```python
from build123d import *

# Parameters (mm, degrees)
RESSALTO_EXTRUS_O1_DEPTH = 6


with BuildPart() as part:
    # Model → Ressalto-extrusão1 (new body)
    with BuildSketch(Plane.XY):
        with BuildLine():
            Line((216.587601096, 108.090872109), (216.587601096, 136.090872109))
            Line((216.587601096, 136.090872109), (166.347707202, 261.690606843))
            ThreePointArc((166.347707202, 261.690606843), (163.772772031, 264.887342722), (159.848370366, 266.090872109))
            Line((159.848370366, 266.090872109), (157.518730442, 266.090872109))
            Line((157.518730442, 266.090872109), (157.518730442, 253.090872109))
            ThreePointArc((157.518730442, 253.090872109), (153.518730442, 249.090872109), (149.518730442, 253.090872109))
            Line((149.518730442, 253.090872109), (149.518730442, 266.090872109))
            Line((149.518730442, 266.090872109), (146.518730442, 266.090872109))
            ThreePointArc((146.518730442, 266.090872109), (141.568982974, 264.040619577), (139.518730442, 259.090872109))
            Line((139.518730442, 259.090872109), (139.518730442, 244.812476299))
            ThreePointArc((139.518730442, 244.812476299), (139.645035735, 243.488723651), (140.019393606, 242.212741564))
            Line((140.019393606, 242.212741564), (182.587601096, 135.792222839))
            Line((182.587601096, 135.792222839), (182.587601096, 88.090872109))
            ThreePointArc((182.587601096, 88.090872109), (184.637853628, 83.141124641), (189.587601096, 81.090872109))
            Line((189.587601096, 81.090872109), (198.587601096, 81.090872109))
            Line((198.587601096, 81.090872109), (198.587601096, 121.090872109))
            Line((198.587601096, 121.090872109), (204.587601096, 121.090872109))
            Line((204.587601096, 121.090872109), (204.587601096, 101.090872109))
            Line((204.587601096, 101.090872109), (209.587601096, 101.090872109))
            ThreePointArc((209.587601096, 101.090872109), (214.537348564, 103.141124641), (216.587601096, 108.090872109))
        make_face()
    extrude(amount=RESSALTO_EXTRUS_O1_DEPTH)


solid = part.part
```
Input: part model. Units: mm. Frame: model coordinates. A direction names the side the tool comes from. Give positions to 0.01 mm unless a question says otherwise; leave off trailing zeros. Loops run counter-clockwise (first coordinate to the right, second up) from the corner with the lowest first, then second, coordinate; pieces in that order, holes last. Notation, with made-up numbers: (52.5, -20.75) -> (86.5, -20.75) arc R25 cw to (86.5, -5.75) -> close; hole circle Ø4 at (-23.75, 79.5). An arc over 180 degrees is marked (long way). Use a Markdown table: item, result.
Q1. Access query for faces 1 (the cylindrical face through (163.821, 264.854, 2.958)), 2 (the flat face through (207, 101.091, 3)), 3 (the flat face through (149.519, 259, 3)), 4 (the flat face through (194, 81.091, 3)), 5 (the flat face through (202, 121.091, 3)). Directions: +Z, -Z, +X, -X, +Y, -Y. A direction counts if a zero-diameter tool reaches every point of the face in a straight line with its end or side. Return the directions, or none.
Entries:
| item | result |
|---|---|
| face 1 | +Z, -Z, +X, +Y |
| face 2 | +Z, -Z, +X, -Y |
| face 3 | +Z, -Z, +Y |
| face 4 | +Z, -Z, +X, -X, -Y |
| face 5 | +Z, -Z, -Y |
Q2. Section query A-A, the plane y = 115. Return the cut outline in (x, z), plus the area to 3 significant figures.
Entries:
| item | result |
|---|---|
| outline | (182.59, 0) -> (198.59, 0) -> (198.59, 6) -> (182.59, 6) -> close; (204.59, 0) -> (216.59, 0) -> (216.59, 6) -> (204.59, 6) -> close |
| area | 168 mm² |
Q3. Pull-direction query (X, two-part tool) for faces 6 (the flat face through (161.006, 189.747, 2.958)), 7 (the flat face through (204.588, 111, 3)), 8 (the flat face through (191.82, 198.01, 2.96)); classes: pulls with the +X half, pulls with the -X half, needs draft (parallel to the pull), parting line crosses it, or undercut.
Entries:
| item | result |
|---|---|
| face 6 | pulls with the -X half |
| face 7 | undercut |
| face 8 | pulls with the +X half |
Q4. Ray query, probe 1 along X at (y, z) = (118, 1.3); probe 2 along X at (y, z) = (253.5, 1.2); probe 3 along Y at (x, z) = (195, 1.3). Return the intervals inside material, ascending. Write a range as from..to.
Entries:
| item | result |
|---|---|
| probe 1 | x = 182.59..198.59, 204.59..216.59 |
| probe 2 | x = 139.52..149.52, 157.52..169.62 |
| probe 3 | y = 81.09..190.06 |
Q5. Section query C-C, the plane x = 207.5. Return the cut outline in (y, z), plus the area to 3 significant figures.
Entries:
| item | result |
|---|---|
| outline | (101.09, 0) -> (158.81, 0) -> (158.81, 6) -> (101.09, 6) -> close |
| area | 346 mm² |
Q6. Section query B-B, the plane z = 3.35. Return the cut outline in (x, y).
Entries:
| item | result |
|---|---|
| outline | (139.52, 244.81) arc R7 ccw to (140.02, 242.21) -> (182.59, 135.79) -> (182.59, 88.09) arc R7 ccw to (189.59, 81.09) -> (198.59, 81.09) -> (198.59, 121.09) -> (204.59, 121.09) -> (204.59, 101.09) -> (209.59, 101.09) arc R7 ccw to (216.59, 108.09) -> (216.59, 136.09) -> (166.35, 261.69) arc R7 ccw to (159.85, 266.09) -> (157.52, 266.09) -> (157.52, 253.09) arc R4 cw to (149.52, 253.09) -> (149.52, 266.09) -> (146.52, 266.09) arc R7 ccw to (139.52, 259.09) -> close |
Q7. First-contact query: P1, Ø3, axis at y = 108.5, z = 2, coming from the -X side; P2, Ø1.5, axis at x = 186.5, z = 2, coming from the -Y side; P3, Ø1, axis at x = 153.5, z = 4, coming from the -Y side. Flat tips, straight axial feed; report the tip coordinate or a pass-through.
Entries:
| item | result |
|---|---|
| P1 | stops at x = 182.59 |
| P2 | stops at y = 81.49 |
| P3 | stops at y = 207.26 |
Q8. Section query D-D, the plane y = 162. Return the cut outline in (x, z), plus the area to 3 significant figures.
Entries:
| item | result |
|---|---|
| outline | (172.1, 0) -> (206.22, 0) -> (206.22, 6) -> (172.1, 6) -> close |
| area | 205 mm² |
